Autodesk Inventor part; units mm, degrees
ref_plane "Piano di lavoro1" through (0, 0, 2) normal (0, 0, -1) x (-1, 0, 0)
ref_plane "YZ Plane" through (0, 0, 0) normal (1, 0, 0) x (0, 1, 0)
ref_plane "XZ Plane" through (0, 0, 0) normal (0, 1, 0) x (-1, 0, 0)
sketch "Schizzo1" plane through (0, 0, 0) normal (0, 0, 1) x (1, 0, 0)
  line L0 (0, 7.5056) -> (6.5, 3.7528)
  line L1 (6.5, 3.7528) -> (6.5, -3.7528)
  line L2 (6.5, -3.7528) -> (0, -7.5056)
  line L3 (0, -7.5056) -> (-6.5, -3.7528)
  line L4 (-6.5, -3.7528) -> (-6.5, 3.7528)
  line L5 (-6.5, 3.7528) -> (0, 7.5056)
  point P0 (0, 0)
  point P1 (0, 0)
  dimension "d0" = 13
extrude "Estrusione1" add sketch "Schizzo1" along normal blind 4
sketch "Schizzo2" plane through (0, 0, 4) normal (0, 0, 1) x (1, 0, 0)
  circle A0 centre (0, 0) radius 5.5
  dimension "d5" = 11
extrude "Estrusione2" add sketch "Schizzo2" along normal blind 1.5
sketch "Schizzo3" plane through (0, 0, 0) normal (1, 0, 0) x (0, 1, 0)
  line L0 (7.5056, 4) -> (3.7528, 4)
  line L1 (3.7528, 0) -> (3.7528, 4)
  line L2 (7.5056, 0) -> (3.7528, 0)
  line L3 (7.5056, 0) -> (7.5056, 4)
  line L4 (6.3093, 0) -> (7.5056, 0.6907)
  line L5 (0, -1) -> (0, 6)
  line L6 (6.3093, 4) -> (7.5056, 4)
  line L7 (6.3093, 4) -> (7.5056, 3.3093)
  point P0 (0, 0)
  dimension "d6" = 30
  dimension "d23" = 30
ref_plane "Piano di lavoro1" through (0, 0, 2) normal (0, 0, -1) x (-1, 0, 0)
sketch "Schizzo4" plane through (0, 0, 5.5) normal (0, 0, 1) x (1, 0, 0)
  circle A0 centre (0, 0) radius 5.5
hole "Foro1" at (0, 0, 5.5) direction (0, 0, -1) diameter 8 end through all
thread "Filettatura1"
chamfer "Smusso1" distance 0.5 angle 45 2 edges at (0, 4, 5.5) (0, 4, 0)
revolve "Rivoluzione2" cut sketch "Schizzo3" angle 360 about axis through (0, 0, -10) along (0, 0, 1) contours L3 L7 L0 | L3 L2 L4
fillet "Raccordo1" radius 0.5 1 edges at (-5.5, 0, 5.5)
properties part number "Dado 13"
Check sheet for the modelled part. Datum: model origin and axes. Units: mm. A direction names the side the tool comes from. Coordinates: 2 decimals unless noted, no trailing zeros. Write each loop counter-clockwise with the first axis right and the second up, starting at its lowest first coordinate (ties: lowest second). Pieces come first, ordered by that corner, then holes. Notation, with made-up numbers: M 40.5,86 L 93.5,86 A19 ccw 93.5,105 Z; hole C 75,33 d9. An arc over 180 degrees is marked long. Answer as CSV lines item,"result".
Q1. Cross-section at A-A (z = 2.1). Record the boundary of the cut face in (x, y), then the cut area to 3 significant figures.
Check result:
outline,"M -6.5,-3.75 L 0,-7.51 L 6.5,-3.75 L 6.5,3.75 L 0,7.51 L -6.5,3.75 Z; hole C 0,0 d8"
area,"96.1 mm^2"
Q2. Mould release check, pull along Y, two halves, no side actions. Record for faces 1 (the face through (-3.2, -5.66, 1.97)), 2 (the face through (3.905, 0.867, 2.718)), 3 (the face through (3.2, 5.66, 1.97)), 4 (the face through (6.5, 0, 2)): released by +Y, released by -Y, zero draft, split by the parting line, or undercut.
Check result:
face 1,"released by -Y"
face 2,"undercut"
face 3,"released by +Y"
face 4,"zero draft"
Q3. Go/stop test with flat-tipped pins: pin 1 (1.5 mm diameter, centred on x = 3, z = 3.5, fed in from -Y); pin 2 (2 mm diameter, centred on y = -4.5, z = 4.5, fed in from -X); pin 3 (5 mm diameter, centred on x = 0, y = 0, fed in from +Z). Record where each tip stops, or that it passes through.
Check result:
pin 1,"y = -6.21"
pin 2,"x = -5.72"
pin 3,"through"
Q4. Material ranges on probe 1 along X at (y, z) = (0, 3.85); probe 2 along Z at (x, y) = (-5.25, -3); probe 3 along X at (y, z) = (-0.75, 1.4), recorded low to high. Write a range as from..to.
Check result:
probe 1,"-6.5..-4, 4..6.5"
probe 2,"0..4"
probe 3,"-6.5..-3.93, 3.93..6.5"
Q5. Set-up check for faces 5 (the face through (3.3, -5.6, 2)), 6 (the face through (-1.19, 5.37, 4.49)): record each of +Z, -Z, +X, -X, +Y, -Y from which the full face is reachable in a straight line by a thin tool's end or side.
Check result:
face 5,"+Z, -Z, +X, -Y"
face 6,"+Z"
Q6. Cross-section at B-B (y = 0). Record the boundary of the cut face in (x, z), then the cut area to 3 significant figures.
Check result:
outline,"M -6.5,0.11 L -6.31,0 L -4.5,0 L -4,0.5 L -4,5 L -4.5,5.5 L -5,5.5 A0.5 ccw -5.5,5 L -5.5,4 L -6.31,4 L -6.5,3.89 Z; M 4,0.5 L 4.5,0 L 6.31,0 L 6.5,0.11 L 6.5,3.89 L 6.31,4 L 5.5,4 L 5.5,5 A0.5 ccw 5,5.5 L 4.5,5.5 L 4,5 Z"
area,"23.9 mm^2"
